Verification items for this drawing (mm, ordinates from the low corner). Round coordinates to 2 decimals unless told otherwise and drop trailing zeros. Loops run counter-clockwise (first coordinate to the right, second up) from the corner with the lowest first, then second, coordinate; pieces in that order, holes last. Notation, with made-up numbers: (50, 19.5) - (63, 19.5) arc R12 cw to (63, 32.5) - close; hole circle Ø6 at (80, -15). An arc over 180 degrees is marked (long way). Put each result on its own line as item: value.
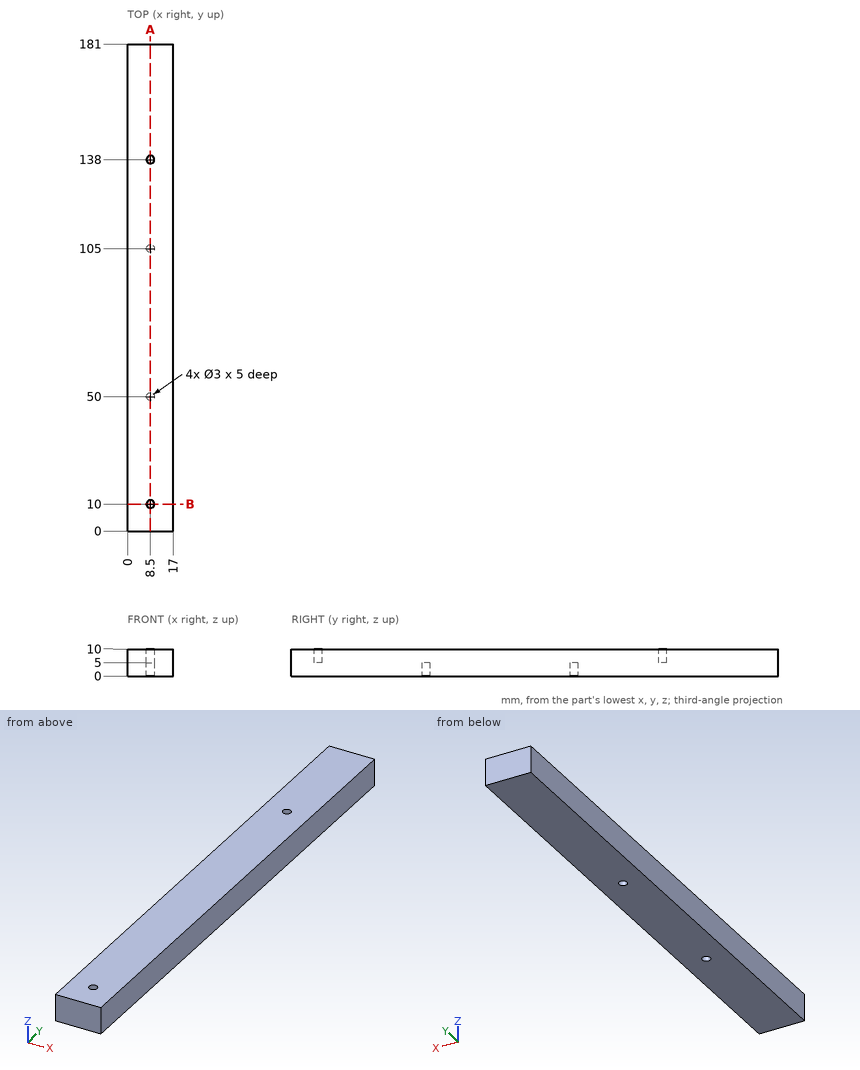
Item 1: Section check B-B on y = 10. Enter the section's corners in (x, z).
Filled sheet:
outline: (0, 0) - (17, 0) - (17, 10) - (10, 10) - (10, 5) - (7, 5) - (7, 10) - (0, 10) - close
Item 2: Go/stop test with a flat-tipped pin: pin 1 (1.5 mm diameter, centred on x = 8, y = 10, fed in from +Z). Record where the tip stops, or that it passes through.
Filled sheet:
pin 1: z = 5
Item 3: Section check A-A on x = 8.5. Enter the section's corners in (y, z).
Filled sheet:
outline: (0, 0) - (48.5, 0) - (48.5, 5) - (51.5, 5) - (51.5, 0) - (103.5, 0) - (103.5, 5) - (106.5, 5) - (106.5, 0) - (181, 0) - (181, 10) - (139.5, 10) - (139.5, 5) - (136.5, 5) - (136.5, 10) - (11.5, 10) - (11.5, 5) - (8.5, 5) - (8.5, 10) - (0, 10) - close
Item 4: Thickness scan on line 1 (Y direction, x = 8.5, z = 8.6); line 2 (Y direction, x = 8.5, z = 3.6); line 3 (X direction, y = 105, z = 1.4). Record the ranges inside material, lowest first. Write a range as from..to.
Filled sheet:
line 1: 0..8.5, 11.5..136.5, 139.5..181
line 2: 0..48.5, 51.5..103.5, 106.5..181
line 3: 0..7, 10..17
